Autodesk Inventor part; units mm, degrees
ref_plane "YZ Plane" through (0, 0, 0) normal (1, 0, 0) x (0, 1, 0)
ref_plane "XZ Plane" through (0, 0, 0) normal (0, 1, 0) x (-1, 0, 0)
ref_plane "XY Plane" through (0, 0, 0) normal (0, 0, 1) x (1, 0, 0)
sketch "Sketch1" plane through (0, 0, 0) normal (0, 0, 1) x (1, 0, 0)
  circle A0 centre (0, 0) radius 2.159
  dimension "d0" = 4.318
extrude "Extrusion1" add sketch "Sketch1" along normal blind 10.16
sketch "Sketch2" plane through (0, 0, 0) normal (0, 0, -1) x (-1, 0, 0)
  circle A0 centre (0, 0) radius 2.159
  circle A1 centre (0, 0) radius 1.4986
  dimension "d3" = 2.9972
extrude "Extrusion2" cut sketch "Sketch2" against normal blind 6.096
sketch "Sketch3" plane through (0, 0, 0) normal (0, 0, -1) x (-1, 0, 0)
  circle A0 centre (0, 0) radius 1.4986
hole "Hole1" at (0, 0, 0) direction (0, 0, 1) diameter 1.7272 end through all
chamfer "Chamfer1" distance 0.635 angle 45 1 edges at (-2.159, 0, 10.16)
properties part number "Connector"
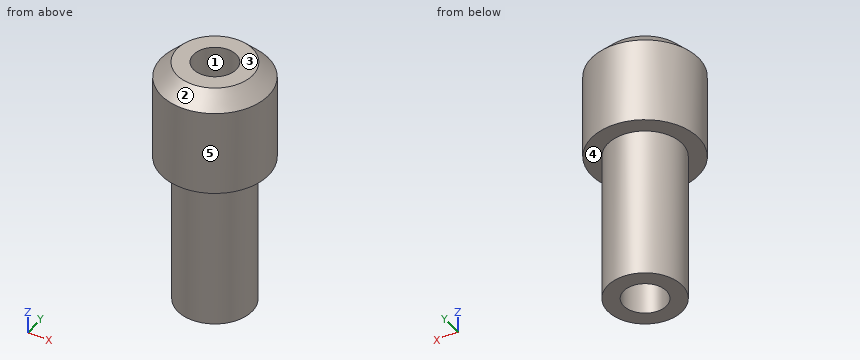
The listing builds one solid part. Answer for the finished solid, in the listing's coordinates (mm). Face numbers are marked on the shaded views. A direction names the side the tool comes from. Give positions to 0.01 mm unless a question says otherwise; leave off trailing zeros. Order: outer loops, then holes, each group sorted by start corner. A loop starts at its lowest first (then second) coordinate and runs counter-clockwise, first axis right, second up. Notation, with made-up numbers: M -6.75,71 L 45.25,71 A27 cw 45.25,105 Z; hole C 68,82 d4. An arc over 180 degrees is marked long. Put each result on its own line as item: value. Start each with the question number.
Item 1: For a pull along X with two mould halves and no side action, classify the marked faces 1, 2 and 3 as +X half, -X half, draft (parallel to the pull), parting line (faces both ways), or undercut.
Item 2: Which of the six approach directions +Z, -Z, +X, -X, +Y, -Y give full straight-line access (tool end or side, diameter ignored) to the marked faces 4 and 5?
Item 3: Find the intervals of material crossed by line 1 along Y through (x, z) = (0, 8); line 2 along X through (y, z) = (-0.65, 5.75), in increasing order.
Item 4: The part is cut by section D-D, the plane z = 8.25. Determine the outline of the cut face in (x, y).
Item 5: The part is cut by section C-C, the plane z = 3. Determine the outline of the cut face in (x, y).
Item 6: The part is cut by section A-A, the plane y = 0. Determine the outline of the cut face in (x, z) (3 decimals), and give its area (3 significant figures).
Item 7: Flat-ended cylindrical pins translate along their axes: P1, Ø1, axis at y = 1, z = 5, coming from the +X side; P2, Ø2, axis at y = 0, z = 4, coming from the +X side; P3, Ø1.5, axis at x = 0.5, y = -1.5, coming from the -Z side; P4, Ø2, axis at x = -1, z = 2.5, coming from the +Y side. Find the tip coordinate at first contact, or state that the pin passes through.
Answer key:
1. face 1: undercut
1. face 2: parting line
1. face 3: draft
2. face 4: -Z
2. face 5: +Z, -Z
3. line 1: y = -2.16 to -0.86, 0.86 to 2.16
3. line 2: x = -1.35 to -0.57, 0.57 to 1.35
4. outline: C 0,0 d4.32; hole C 0,0 d1.73
5. outline: C 0,0 d3; hole C 0,0 d1.73
6. outline: M -2.159,6.096 L -1.499,6.096 L -1.499,0 L -0.864,0 L -0.864,10.16 L -1.524,10.16 L -2.159,9.525 Z; M 0.864,0 L 1.499,0 L 1.499,6.096 L 2.159,6.096 L 2.159,9.525 L 1.524,10.16 L 0.864,10.16 Z
6. area: 17.9 mm²
7. P1: stops at x = 1.41
7. P2: stops at x = 1.5
7. P3: stops at z = 0
7. P4: stops at y = 1.5
